Here's how the part is built. I have some questions about the finished solid (model axes, mm). Round coordinates to 2 decimals unless told otherwise and drop trailing zeros. Write each loop counter-clockwise with the first axis right and the second up, starting at its lowest first coordinate (ties: lowest second). Pieces come first, ordered by that corner, then holes. Notation, with made-up numbers: M -21.5,8 L 4.5,8 A30 cw 4.5,42 Z; hole C -24.75,29.25 d7. An arc over 180 degrees is marked long. Use a Markdown table: item, result. Add a question column.
```python
from build123d import *

# Parameters (mm, degrees)
SKETCH1_W                  = 323.85
SKETCH1_H                  = 127
BOSS_EXTRUDE1_DEPTH        = 3.175
SKETCH2_R                  = 6.35
SKETCH2_W                  = 12.7
SKETCH2_H                  = 19.05
CUT_EXTRUDE1_DEPTH         = 4.175
F_10_CLEARANCE_HOLE1_D     = 5.1054
F_10_CLEARANCE_HOLE1_DEPTH = 12.7
F_10_CLEARANCE_HOLE1_TIP   = 1.533816902


with BuildPart() as part:
    # Sketch1 → Boss-Extrude1 (new body)
    with BuildSketch(Plane(origin=(0, 0, 0), x_dir=(1, 0, 0), z_dir=(0, 1, 0))):
        with Locations((161.925, 63.5)):
            Rectangle(SKETCH1_W, SKETCH1_H)
    extrude(amount=BOSS_EXTRUDE1_DEPTH)

    # Sketch2 → Cut-Extrude1 (cut, through all)
    with BuildSketch(Plane(origin=(0, 0, 0), x_dir=(-1, 0, 0), z_dir=(0, -1, 0))):
        with Locations((-41.275, 112.649)):
            Circle(SKETCH2_R)
        with Locations((-25.4, 19.05)):
            Circle(SKETCH2_R)
        with Locations((-25.4, 9.525)):
            Rectangle(SKETCH2_W, SKETCH2_H)
    extrude(amount=-CUT_EXTRUDE1_DEPTH, mode=Mode.SUBTRACT)

    # #10 Clearance Hole1
    with Locations(Plane(origin=(0, 0, 0), x_dir=(-1, 0, 0), z_dir=(0, -1, 0))):
        with Locations((-315.9125, 70.75), (-315.9125, 56.25), (-7.9375, 70.75), (-7.9375, 56.25)):
            Hole(F_10_CLEARANCE_HOLE1_D / 2, depth=F_10_CLEARANCE_HOLE1_DEPTH)
            with Locations((0, 0, -(F_10_CLEARANCE_HOLE1_DEPTH + F_10_CLEARANCE_HOLE1_TIP / 2))):  # 118° drill point
                Cone(0, F_10_CLEARANCE_HOLE1_D / 2, F_10_CLEARANCE_HOLE1_TIP, mode=Mode.SUBTRACT)


solid = part.part
```
Item 1: Imagine slicing it at A-A on x = 25.4. List the corners of the cut face in (y, z) for me (3 decimals).
Item 2: For pin 1 Ø3 at (x, z) = (246, -70) entering from -Y, with a flat end and sliding along its axis, tell me the tip position at first contact or that it passes through.
Item 3: If we mould it in two halves opening along Z, with no side actions, what happens to faces 1 (the face through (47.62, 1.57, -112.93)), 2 (the face through (160, 3.175, -64)), 3 (the face through (25.3, 1.6, -25.4))? For each: +Z half, -Z half, draft (parallel to the pull), parting line (faces both ways), or undercut.
Item 4: I need wall thicknesses on probe 1 along X at (y, z) = (0.7, -56.25); probe 2 along X at (y, z) = (2.1, -19.5); probe 3 along X at (y, z) = (2.25, -69). Which ranges of each line are inside material? Lowest first, please. Write a range as from..to.
The answers:
| question | item | result |
|---|---|---|
| 1 | outline | M 0,-127 L 3.175,-127 L 3.175,-25.4 L 0,-25.4 Z |
| 2 | pin 1 | y = 0 |
| 3 | face 1 | undercut |
| 3 | face 2 | draft |
| 3 | face 3 | +Z half |
| 4 | probe 1 | 0..5.38, 10.49..313.36, 318.47..323.85 |
| 4 | probe 2 | 0..19.07, 31.73..323.85 |
| 4 | probe 3 | 0..6.08, 9.8..314.05, 317.77..323.85 |
